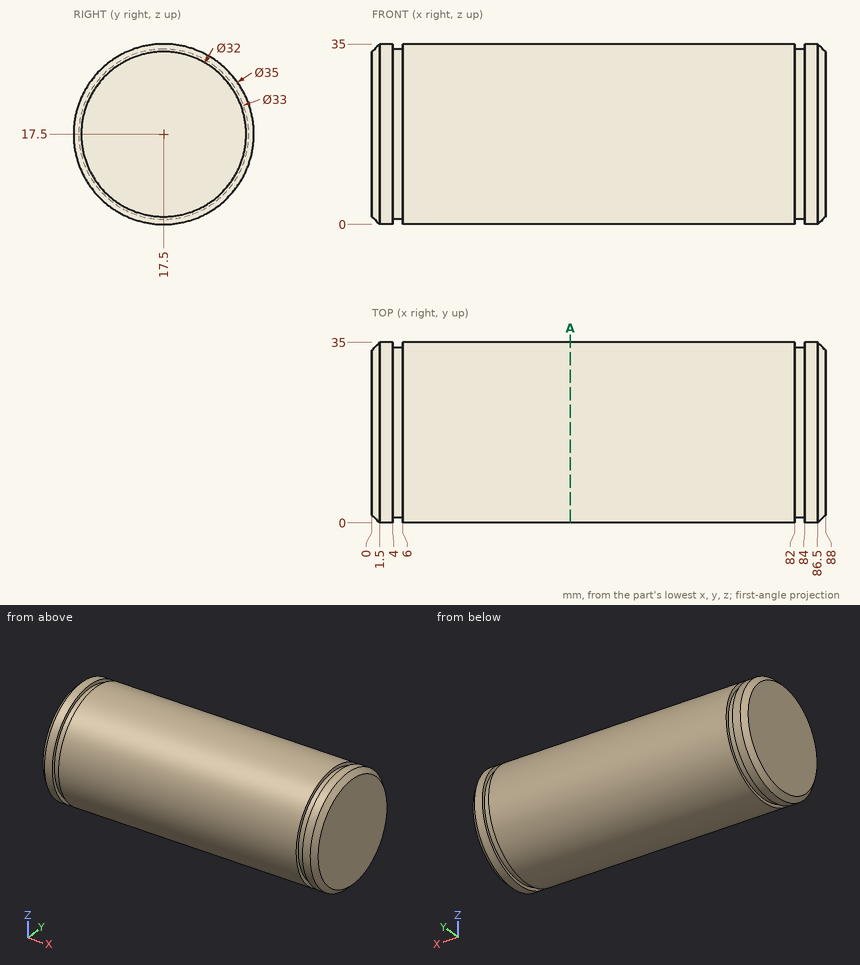
Here's the drawing with two shaded views (mm, measured from the low corner). I have some questions. Give positions to 0.01 mm unless a question says otherwise; leave off trailing zeros. Write each loop counter-clockwise with the first axis right and the second up, starting at its lowest first coordinate (ties: lowest second). Pieces come first, ordered by that corner, then holes. Notation, with made-up numbers: (18, 23.5) -> (65, 23.5) arc R22 ccw to (65, 31.5) -> close; hole circle Ø7 at (-19.75, -10). An arc over 180 degrees is marked (long way). One line per item, written item: value.
Q1. Please list where these lines run through material, in increasing order: line 1 (X direction, y = 29.5, z = 5); line 2 (Y direction, x = 34.5, z = 18); line 3 (Z direction, x = 40, y = 29). Write a range as [from, to].
Results found:
line 1: x = [1.33, 4], [6, 82], [84, 86.67]
line 2: y = [0.01, 34.99]
line 3: z = [4.31, 30.69]
Q2. For P1, Ø3, axis at x = 54.5, y = 21, coming from the -Z side; P2, Ø3, axis at x = 15, y = 6, coming from the +Z side; P3, Ø5, axis at x = 44.5, z = 25, coming from the +Y side; P4, Ø10.5, axis at y = 15, z = 26, coming from the -X side, each with a flat end and sliding along its axis, tell me the tip position at first contact or that it passes through.
Results found:
P1: stops at z = 0.11
P2: stops at z = 31.86
P3: stops at y = 34.27
P4: stops at x = 0
Q3. Imagine slicing it at A-A on x = 38.5. Please give me the cut outline in (y, z).
Results found:
outline: circle Ø35 at (17.5, 17.5)
